Check sheet for the modelled part. Datum: model origin and axes. Units: mm. A direction names the side the tool comes from. Coordinates: 2 decimals unless noted, no trailing zeros. Write each loop counter-clockwise with the first axis right and the second up, starting at its lowest first coordinate (ties: lowest second). Pieces come first, ordered by that corner, then holes. Notation, with made-up numbers: (59, 23) - (104, 23) arc R10 ccw to (104, 27) - close; hole circle Ø8 at (50, 50.5). An arc over 180 degrees is marked (long way). Use one line per item in the form item = value. Start each with the question number.
1. Tool access check on faces 1 (the face through (0, 3, -18.915)), 2 (the face through (-5, 6, -64)), 3 (the face through (-0.1, 1, -14.6)), 4 (the face through (7, -4, -22)). Record the directions out of +Z, -Z, +X, -X, +Y, -Y that give a thin tool (end or side, any length) a straight path to the whole face; none if there is none.
2. Draft check along X on faces 5 (the face through (7.54, 0.4, -49.81)), 6 (the face through (-0.09, 1, -46.23)), 7 (the face through (0, 5, -14)). Enter one of: +X half, -X half, draft (parallel to the pull), parting line (faces both ways), or undercut.
3. Cross-section at A-A on x = 0. Give the number of separate pieces and of enclosed holes in the cut face, then the cut area to 3 significant figures.
4. Go/stop test with flat-tipped pins: pin 1 Ø4.5 at (x, y) = (-1.5, 2.5) entering from -Z; pin 2 Ø1.8 at (x, z) = (0.5, -46) entering from -Y; pin 3 Ø1.5 at (x, z) = (5, -11.5) entering from +Y; pin 4 Ø2.5 at (y, z) = (8.09, -70.49) entering from -X. Record where each tip stops, or that it passes through.
5. Cross-section at B-B on z = -38.5. Record the boundary of the cut face in (x, y).
6. Scan lines: line 1 along X through (y, z) = (3.5, 0); line 2 along X through (y, z) = (-3, -36.5); line 3 along Y through (x, z) = (-5.25, -6). Record each from-to range of solid material in increasing order.
7. Cross-section at D-D on z = 4. Record the boundary of the cut face in (x, y).
```python
from build123d import *

# Parameters (mm, degrees)
EXTRUDE_1_DEPTH     = 10
SKETCH_2_R          = 6.7
CUT_EXTRUDE_1_DEPTH = 5
SKETCH_4_R          = 3.2
CUT_EXTRUDE_3_DEPTH = 57.124860802
SKETCH_3_W          = 12.4
SKETCH_3_H          = 23.085257288
CUT_EXTRUDE_2_DEPTH = 57.621550668
SKETCH_5_W          = 12.4
SKETCH_5_H          = 34.914742712
CUT_EXTRUDE_4_DEPTH = 5
SKETCH_6_R          = 1.1
CUT_EXTRUDE_5_DEPTH = 57.124860802
FILLET_1_R          = 8
SKETCH_9_R          = 1.6
EXTRUDE_2_DEPTH     = 5
CHAMFER_2_SIZE      = 5


with BuildPart() as part:
    # 草图1 → 凸台-拉伸1 (new, symmetric)
    with BuildSketch(Plane(origin=(0, 0, 0), x_dir=(0, 0, -1), z_dir=(1, 0, 0))):
        Polygon((55, -4), (50.256311045, 5), (-10, 5), (-10, -4), align=None)
    extrude(amount=EXTRUDE_1_DEPTH, both=True)

    # 草图2 → 切除-拉伸1 (cut)
    with BuildSketch(Plane(origin=(0, -4, 0), x_dir=(1, 0, 0), z_dir=(0, 1, 0))):
        with Locations(Location((0, 0, 0), (0, 0, 270))):
            Circle(SKETCH_2_R)
    extrude(amount=CUT_EXTRUDE_1_DEPTH, mode=Mode.SUBTRACT)

    # 草图4 → 切除-拉伸3 (cut, through all)
    with BuildSketch(Plane.XZ.offset(-1)):
        with Locations(Location((0, 0, 0), (0, 0, 270))):
            Circle(SKETCH_4_R)
    extrude(amount=-CUT_EXTRUDE_3_DEPTH, mode=Mode.SUBTRACT)

    # 草图3 → 切除-拉伸2 (cut, through all)
    with BuildSketch(Plane(origin=(0, 5, 0), x_dir=(1, 0, 0), z_dir=(0, 1, 0))):
        with Locations((0, 30.457371356)):
            Rectangle(SKETCH_3_W, SKETCH_3_H)
    extrude(amount=-CUT_EXTRUDE_2_DEPTH, mode=Mode.SUBTRACT)

    # 草图5 → 切除-拉伸4 (cut)
    with BuildSketch(Plane.XZ.offset(4)):
        with Locations((0, -30.457371356)):
            Rectangle(SKETCH_5_W, SKETCH_5_H)
    extrude(amount=-CUT_EXTRUDE_4_DEPTH, mode=Mode.SUBTRACT)

    # 草图6 → 切除-拉伸5 (cut, through all)
    with BuildSketch(Plane.XZ.offset(-1)):
        with Locations(Location((0, -15.957371356, 0), (0, 0, 270))):
            Circle(SKETCH_6_R)
        with Locations(Location((0, -44.957371356, 0), (0, 0, 90))):
            Circle(SKETCH_6_R)
    extrude(amount=-CUT_EXTRUDE_5_DEPTH, mode=Mode.SUBTRACT)

    # 圆角1
    fillet_1_edges = [part.edges().sort_by_distance(p)[0] for p in [
        (10, 0.5, 10),
        (-10, 0.5, 10),
    ]]
    fillet(fillet_1_edges, radius=FILLET_1_R)

    # 草图9 → 凸台-拉伸2 (add, symmetric)
    with BuildSketch(Plane(origin=(0, 0, 0), x_dir=(0, 0, -1), z_dir=(1, 0, 0))):
        Polygon((55, -4), (77.512583876, 5.666104035), (73.567235291, 14.85491378), (50.614909072, 5), (50.256311045, 5), align=None)
        with Locations((70.486064224, 8.090567185)):
            Circle(SKETCH_9_R, mode=Mode.SUBTRACT)
        with Locations((58.540611554, 2.961614024)):
            Circle(SKETCH_9_R, mode=Mode.SUBTRACT)
    extrude(amount=EXTRUDE_2_DEPTH, both=True)

    # 倒角2
    chamfer_2_edges = [part.edges().sort_by_distance(p)[0] for p in [
        (-10, 0.5, -52.628155522),
        (10, 0.5, -52.628155522),
    ]]
    chamfer(chamfer_2_edges, length=CHAMFER_2_SIZE - 0.0001)  # a hair under: the kernel refuses the full size


solid = part.part
```
Final values:
q1.face_1 = +Y, -Y
q1.face_2 = -Z, -X, +Y
q1.face_3 = -Y
q1.face_4 = +Z, -Z, +X, -X, -Y
q2.face_5 = +X half
q2.face_6 = undercut
q2.face_7 = draft
q3.separate_pieces = 5
q3.enclosed_holes = 2
q3.area = 419 mm²
q4.pin_1 = -75.38
q4.pin_2 = 1
q4.pin_3 = 5
q4.pin_4 = through
q5.outline = (-10, -4) - (-6.2, -4) - (-6.2, 5) - (-10, 5) - close; (6.2, -4) - (10, -4) - (10, 5) - (6.2, 5) - close
q6.line_1 = -10 to -3.2, 3.2 to 10
q6.line_2 = -10 to -6.2, 6.2 to 10
q6.line_3 = -4 to 5
q7.outline = (-9.75, -4) - (-5.37, -4) - (-5.37, 1) - (5.37, 1) - (5.37, -4) - (9.75, -4) - (9.75, 5) - (-9.75, 5) - close
